from build123d import *

# Parameters (mm, degrees)
SKETCH1_R          = 1.3
SKETCH1_R_2        = 4.15
EXTRUDE1_DEPTH     = 5.5
EXTRUDE2_DEPTH     = 2.5
FILLET1_R          = 0.5
CUT_EXTRUDE1_DEPTH = 0.5


with BuildPart() as part:
    # Sketch1 → Extrude1 (new body)
    with BuildSketch(Plane.XY):
        with BuildLine():
            Line((35.5, 5.8), (36.8, 5.8))
            Line((36.8, 5.8), (36.8, -5.8))
            Line((36.8, -5.8), (35.5, -5.8))
            Line((35.5, -5.8), (35.5, -13.05))
            Line((35.5, -13.05), (-3.00020865, -13.05))
            Line((-3.00020865, -13.05), (-6.99642445, -2.701859528))
            ThreePointArc((-6.99642445, -2.701859528), (-7.5, 0), (-6.99642445, 2.701859528))
            Line((-6.99642445, 2.701859528), (-3.00020865, 13.05))
            Line((-3.00020865, 13.05), (35.5, 13.05))
            Line((35.5, 13.05), (35.5, 5.8))
        make_face()
        with Locations((31.8, 9.2)):
            Circle(SKETCH1_R, mode=Mode.SUBTRACT)
        with Locations(Location((31.8, -9.2, 0), (0, 0, 180))):
            Circle(SKETCH1_R, mode=Mode.SUBTRACT)
        Circle(SKETCH1_R_2, mode=Mode.SUBTRACT)
    extrude(amount=EXTRUDE1_DEPTH)

    # Sketch2 → Extrude2 (add)
    with BuildSketch(Plane.XY.offset(5.5)):
        with BuildLine():
            Line((7.5, 10), (29.8, 10))
            Line((29.8, 10), (29.8, 9.2))
            ThreePointArc((29.8, 9.2), (30.385786438, 7.785786438), (31.8, 7.2))
            Line((31.8, 7.2), (32.6, 7.2))
            Line((32.6, 7.2), (32.6, -7.2))
            Line((32.6, -7.2), (31.8, -7.2))
            ThreePointArc((31.8, -7.2), (30.385786438, -7.785786438), (29.8, -9.2))
            Line((29.8, -9.2), (29.8, -10))
            Line((29.8, -10), (7.5, -10))
            Line((7.5, -10), (7.5, -8.717797887))
            ThreePointArc((7.5, -8.717797887), (11.5, 0), (7.5, 8.717797887))
            Line((7.5, 8.717797887), (7.5, 10))
        make_face()
    extrude(amount=EXTRUDE2_DEPTH)

    # Fillet1
    fillet1_edges = [part.edges().sort_by_distance(p)[0] for p in [
        (30.385786438, -7.785786438, 8),
        (32.2, -7.2, 8),
        (32.6, 0, 8),
        (32.2, 7.2, 8),
        (30.385786438, 7.785786438, 8),
        (29.8, 9.6, 8),
        (18.65, 10, 8),
        (7.5, 9.358898944, 8),
        (11.5, 0, 8),
        (7.5, -9.358898944, 8),
        (18.65, -10, 8),
        (29.8, -9.6, 8),
    ]]
    fillet(fillet1_edges, radius=FILLET1_R)

    # Sketch3 → Cut-Extrude1 (cut)
    with BuildSketch(Plane.XY.offset(5.5)):
        Polygon((-4.178049077, -10), (35.5, -10), (35.5, -13.05), (-3.00020865, -13.05), align=None)
        Polygon((-4.178049077, 10), (35.5, 10), (35.5, 13.05), (-3.00020865, 13.05), align=None)
    extrude(amount=-CUT_EXTRUDE1_DEPTH, mode=Mode.SUBTRACT)


solid = part.part
Build history of the part. All positions in model axes, mm. A direction names the side the tool comes from. Round coordinates to 2 decimals unless told otherwise and drop trailing zeros. Write each loop counter-clockwise with the first axis right and the second up, starting at its lowest first coordinate (ties: lowest second). Pieces come first, ordered by that corner, then holes. Notation, with made-up numbers: (47.25, 86) - (88.25, 86) arc R11 ccw to (88.25, 95) - close; hole circle Ø6 at (-11.5, 18). An arc over 180 degrees is marked (long way). One line per question, with ' | ' between items.
1. Band-saw the part on A-A, the plane z = 3.5. Write the cut outline in (x, y).
Results are:
outline: (-7, -2.7) - (-3, -13.05) - (35.5, -13.05) - (35.5, -5.8) - (36.8, -5.8) - (36.8, 5.8) - (35.5, 5.8) - (35.5, 13.05) - (-3, 13.05) - (-7, 2.7) arc R7.5 ccw to start; hole circle Ø8.3 at (0, 0); hole circle Ø2.6 at (31.8, -9.2); hole circle Ø2.6 at (31.8, 9.2)
2. Band-saw the part on C-C, the plane x = 25. Write the cut outline in (y, z).
Results are:
outline: (-13.05, 0) - (13.05, 0) - (13.05, 5) - (10, 5) - (10, 7.5) arc R0.5 ccw to (9.5, 8) - (-9.5, 8) arc R0.5 ccw to (-10, 7.5) - (-10, 5) - (-13.05, 5) - close
3. Tool access for faces 1 (the face through (30.4, -7.77, 6.49)), 2 (the face through (36, -5.8, 3)), 3 (the face through (29.8, 9.6, 6.5)): list every direction of +Z, -Z, +X, -X, +Y, -Y with a clear straight run to the whole face (end or side of a thin tool).
Results are:
face 1: +Z, +X, -Y | face 2: +Z, -Z, +X, -Y | face 3: +Z, +X, +Y
4. Band-saw the part on D-D, the plane z = 6. Write the cut outline in (x, y), and give its area (3 significant figures).
Results are:
outline: (7.5, -10) - (29.8, -10) - (29.8, -9.2) arc R2 cw to (31.8, -7.2) - (32.6, -7.2) - (32.6, 7.2) - (31.8, 7.2) arc R2 cw to (29.8, 9.2) - (29.8, 10) - (7.5, 10) - (7.5, 8.72) arc R11.5 cw to (7.5, -8.72) - close | area: 440 mm^2
5. Drop flat-ended pins along their axis: pin 1 Ø2 at (y, z) = (-3.5, 5) entering from -X; pin 2 Ø3.5 at (x, y) = (22, 11.5) entering from +Z; pin 3 Ø1.2 at (x, z) = (13.5, 6.5) entering from +Y; pin 4 Ø6.5 at (x, y) = (0, 0) entering from -Z. Give the stop position or say it passes through.
Results are:
pin 1: x = -7.07 | pin 2: z = 7.93 | pin 3: y = 10 | pin 4: through
6. Mould opens along Y. For faces 4 (the face through (16, -12, 5)), 5 (the face through (32, 7.2, 6)), 6 (the face through (4, -2, 5.5)), 7 (the face through (11.5, -0.1, 6.5)) say: released by +Y, released by -Y, zero draft, split by the parting line, or undercut.
Results are:
face 4: zero draft | face 5: released by +Y | face 6: undercut | face 7: undercut
7. Band-saw the part on B-B, the plane x = 0. Write the cut outline in (y, z).
Results are:
outline: (-13.05, 0) - (-4.15, 0) - (-4.15, 5.5) - (-10, 5.5) - (-10, 5) - (-13.05, 5) - close; (4.15, 0) - (13.05, 0) - (13.05, 5) - (10, 5) - (10, 5.5) - (4.15, 5.5) - close
8. Drill centre lines: line 1 along Y through (x, z) = (31.8, 3.9); line 2 along Y through (x, z) = (0, 1.55); line 3 along Z through (x, y) = (16.5, -11.25). Where is each one in solid material? Low to high. Write a range as from..to.
Results are:
line 1: -13.05..-10.5, -7.9..7.9, 10.5..13.05 | line 2: -13.05..-4.15, 4.15..13.05 | line 3: 0..5
